Build history of the part. All positions in model axes, mm. Give positions to 0.01 mm unless a question says otherwise; leave off trailing zeros. Loops run counter-clockwise (first coordinate to the right, second up) from the corner with the lowest first, then second, coordinate; pieces in that order, holes last. Notation, with made-up numbers: M 59.5,-21 L 77.5,-21 A12 cw 77.5,0 Z; hole C 68,82 d6. An arc over 180 degrees is marked long. Put each result on its own line as item: value.
```python
from build123d import *

# Parameters (mm, degrees)
F1_DEPTH = 3.175


with BuildPart() as f1:
    # F0 (on Top) → F1 (new body)
    with BuildSketch(Plane.XY):
        with BuildLine():
            Line((3.175, 63.5), (-22.225, 63.5))
            Line((-22.225, 63.5), (-22.225, 60.325))
            Line((-22.225, 60.325), (-34.925, 60.325))
            Line((-34.925, 60.325), (-34.925, 12.7))
            Line((-34.925, 12.7), (-38.1, 12.7))
            Line((-38.1, 12.7), (-38.1, -12.7))
            Line((-38.1, -12.7), (-34.925, -12.7))
            Line((-34.925, -12.7), (-34.925, -60.325))
            Line((-34.925, -60.325), (-34.925, -63.5))
            ThreePointArc((-34.925, -63.5), (5.716612, -6.148907), (28.576396, 60.321527))
            Line((28.576396, 60.321527), (3.175, 60.321527))
            Line((3.175, 60.321527), (3.175, 63.5))
        make_face()
    extrude(amount=F1_DEPTH)


solid = f1.part
```
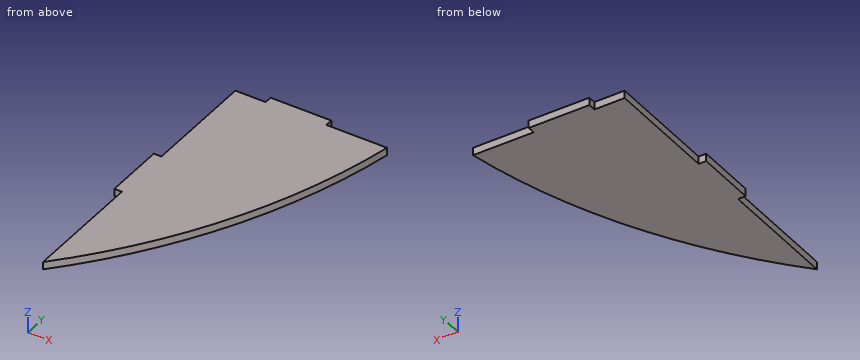
Q1. Slice it at C-C (x = 5). List the corners of the cut face in (y, z) (3 decimals).
Here are the results:
outline: M -7.535,0 L 60.322,0 L 60.322,3.175 L -7.535,3.175 Z
Q2. Drop flat-ended pins along their axis: pin 1 Ø1.6 at (x, z) = (12, 1) entering from +Y; pin 2 Ø1.6 at (y, z) = (33, 1.5) entering from -X (3 decimals); pin 3 Ø1 at (y, z) = (62, 2) entering from +X (3 decimals). Give the stop position or say it passes through.
Here are the results:
pin 1: y = 60.32
pin 2: x = -34.925
pin 3: x = 3.175
Q3. Probe line 1 (X direction, y = -55.5, z = 1.85) (3 decimals); line 2 (Y direction, x = 13, z = 2.85); line 3 (Y direction, x = -8, z = 2.65). List the from-to ranges inside material, lowest first. Write a range as from..to.
Here are the results:
line 1: -34.925..-27.66
line 2: 9.35..60.32
line 3: -29.62..63.5
Q4. Slice it at B-B (y = 30). List the corners of the cut face in (x, z) (3 decimals).
Here are the results:
outline: M -34.925,0 L 20.771,0 L 20.771,3.175 L -34.925,3.175 Z
Q5. Slice it at A-A (z = 0.6). List the corners of the cut face in (x, y) (3 decimals).
Here are the results:
outline: M -38.1,-12.7 L -34.925,-12.7 L -34.925,-63.5 A247.244 ccw 28.576,60.322 L 3.175,60.322 L 3.175,63.5 L -22.225,63.5 L -22.225,60.325 L -34.925,60.325 L -34.925,12.7 L -38.1,12.7 Z
